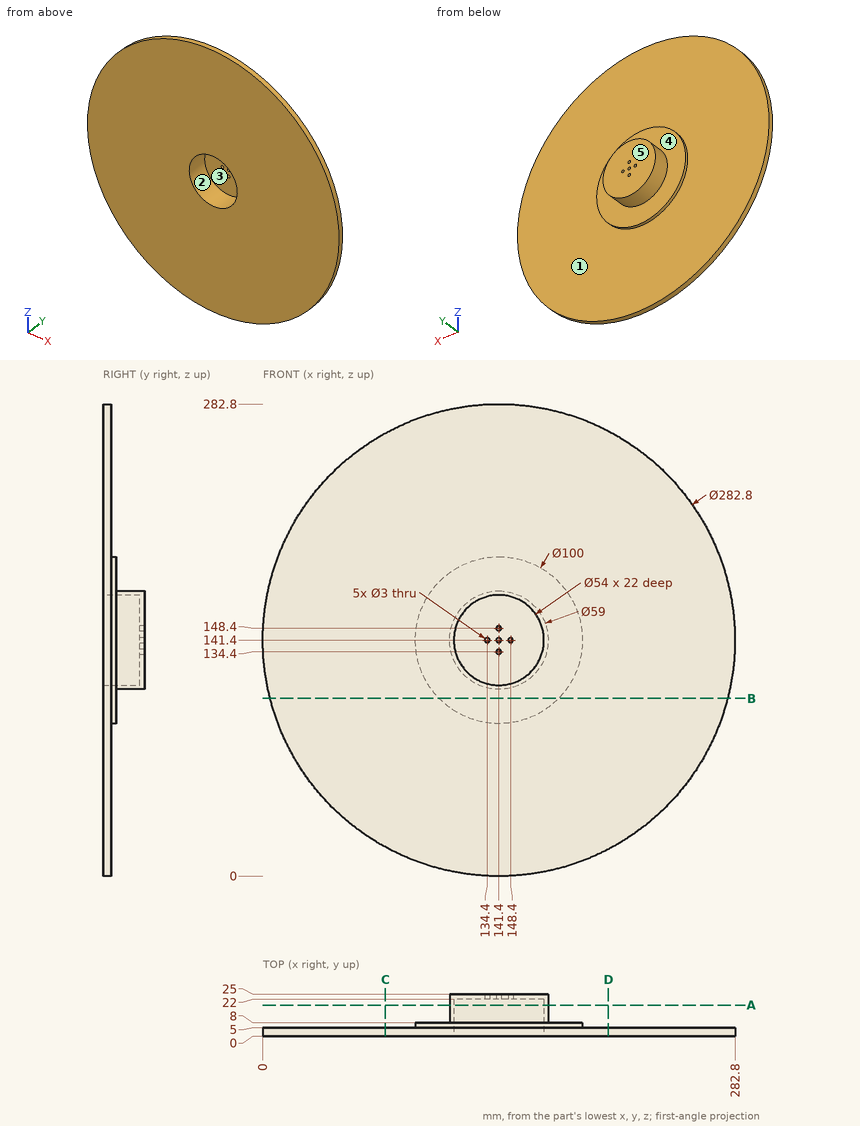
Source: three-view drawing plus pictorial views. Frame: mm from the lowest corner of the part. A direction names the side the tool comes from. Coordinates: 2 decimals unless noted, no trailing zeros. Write each loop counter-clockwise with the first axis right and the second up, starting at its lowest first coordinate (ties: lowest second). Pieces come first, ordered by that corner, then holes. Notation, with made-up numbers: (54.25, 41) - (113.25, 41) arc R28 ccw to (113.25, 74) - close; hole circle Ø9 at (44, -26.75). An arc over 180 degrees is marked (long way). Answer as a JSON object with one key per item and string values.
Q1. Section query C-C, the plane x = 73.5. Output: boundary loops of the cut face in (y, z).
Ans:
{"outline": "(0, 17.37) - (5, 17.37) - (5, 265.43) - (0, 265.43) - close"}
Q2. Section query A-A, the plane y = 18.5. Output: boundary loops of the cut face in (x, z), plus the area to 3 significant figures.
Ans:
{"outline": "circle Ø59 at (141.4, 141.4); hole circle Ø54 at (141.4, 141.4)", "area": "444 mm2"}
Q3. First-contact query: pin 1 Ø1 at (x, z) = (182, 196) entering from +Y; pin 2 Ø5 at (x, z) = (141.4, 148.4) entering from -Y; pin 3 Ø4 at (x, z) = (99.5, 130) entering from +Y. Flat tips, straight axial feed; report the tip coordinate or a pass-through.
Ans:
{"pin 1": "stops at y = 5", "pin 2": "stops at y = 22", "pin 3": "stops at y = 8"}
Q4. Material intervals for line 1 (X direction, y = 15.25, z = 141.4); line 2 (X direction, y = 23.75, z = 141.4); line 3 (X direction, y = 7.25, z = 141.4), sorted ascending. Write a range as [from, to].
Ans:
{"line 1": "x = [111.9, 114.4], [168.4, 170.9]", "line 2": "x = [111.9, 132.9], [135.9, 139.9], [142.9, 146.9], [149.9, 170.9]", "line 3": "x = [91.4, 114.4], [168.4, 191.4]"}
Q5. Set-up query: the marked faces 4 and 5. Return all of +Z, -Z, +X, -X, +Y, -Y with unobstructed straight access to the full face (end or side cutting, diameter ignored); none if empty.
Ans:
{"face 4": "+Y", "face 5": "+Z, -Z, +X, -X, +Y"}
Q6. Section query D-D, the plane x = 207. Output: boundary loops of the cut face in (y, z).
Ans:
{"outline": "(0, 16.14) - (5, 16.14) - (5, 266.66) - (0, 266.66) - close"}
Q7. Section query B-B, the plane z = 106.5. Output: boundary loops of the cut face in (x, y).
Ans:
{"outline": "(4.37, 0) - (278.43, 0) - (278.43, 5) - (177.2, 5) - (177.2, 8) - (105.6, 8) - (105.6, 5) - (4.37, 5) - close"}
Q8. Draft query along X for the marked faces 1, 2 and 3. Return one class per face: released by +X, released by -X, zero draft, split by the parting line, or undercut.
Ans:
{"face 1": "zero draft", "face 2": "undercut", "face 3": "undercut"}
